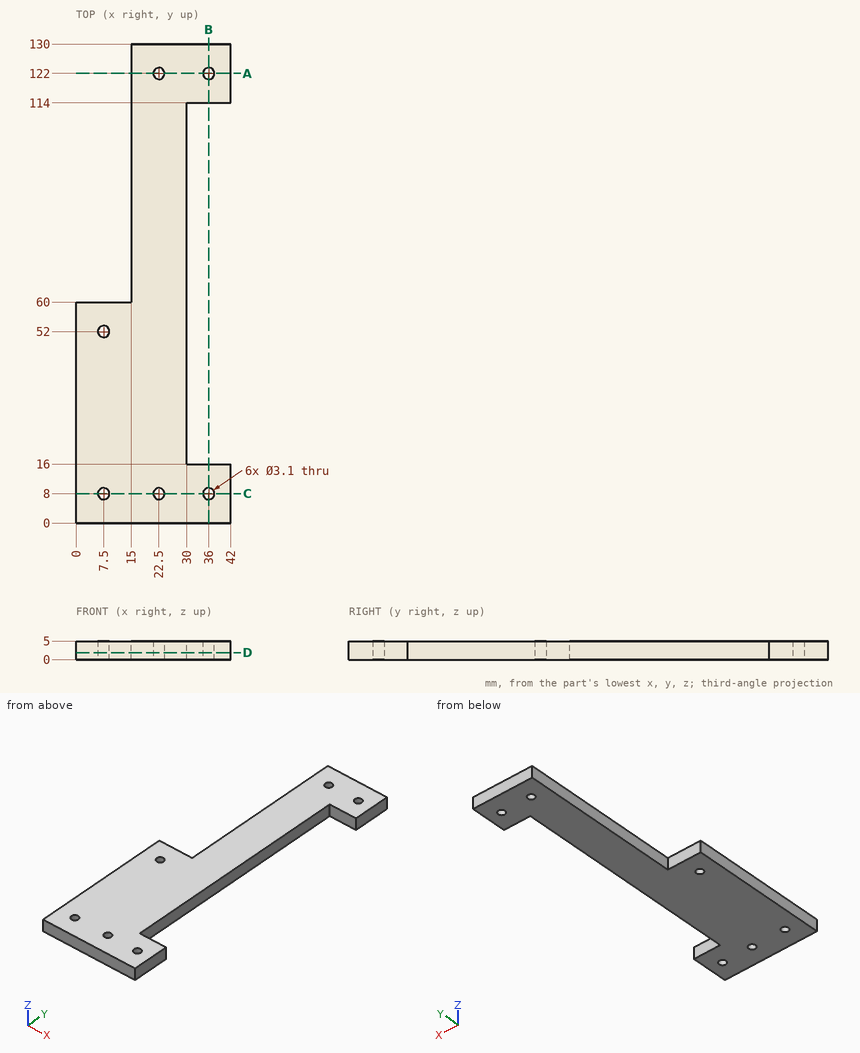
Design review of the part shown in the three views and the two pictorial views. Dimensions are in mm from the part's minimum x, y and z. Coordinates: 2 decimals unless noted, no trailing zeros. Write each loop counter-clockwise with the first axis right and the second up, starting at its lowest first coordinate (ties: lowest second). Pieces come first, ordered by that corner, then holes.
1) We need section B-B on x = 36. State the section outline as (y, z) points, then the cut area to 3 significant figures.
2) We need section C-C on y = 8. State the section outline as (x, z) points, then the cut area to 4 significant figures.
3) To check wall thickness, follow probe 1 along Y at (x, z) = (7.5, 2.15); probe 2 along Y at (x, z) = (22.5, 1.05); probe 3 along Y at (x, z) = (36, 3.8). State the ranges of each line that lie inside material, in increasing order.
4) We need section A-A on y = 122. State the section outline as (x, z) points, then the cut area to 3 significant figures.
5) We need section D-D on z = 1.9. State the section outline as (x, y) points, then the cut area to 3 significant figures.
Answer list:
1. outline: (0, 0) - (6.45, 0) - (6.45, 5) - (0, 5) - close; (9.55, 0) - (16, 0) - (16, 5) - (9.55, 5) - close; (114, 0) - (120.45, 0) - (120.45, 5) - (114, 5) - close; (123.55, 0) - (130, 0) - (130, 5) - (123.55, 5) - close
1. area: 129 mm2
2. outline: (0, 0) - (5.95, 0) - (5.95, 5) - (0, 5) - close; (9.05, 0) - (20.95, 0) - (20.95, 5) - (9.05, 5) - close; (24.05, 0) - (34.45, 0) - (34.45, 5) - (24.05, 5) - close; (37.55, 0) - (42, 0) - (42, 5) - (37.55, 5) - close
2. area: 163.5 mm2
3. probe 1: y = 0 to 6.45, 9.55 to 50.45, 53.55 to 60
3. probe 2: y = 0 to 6.45, 9.55 to 120.45, 123.55 to 130
3. probe 3: y = 0 to 6.45, 9.55 to 16, 114 to 120.45, 123.55 to 130
4. outline: (15, 0) - (20.95, 0) - (20.95, 5) - (15, 5) - close; (24.05, 0) - (34.45, 0) - (34.45, 5) - (24.05, 5) - close; (37.55, 0) - (42, 0) - (42, 5) - (37.55, 5) - close
4. area: 104 mm2
5. outline: (0, 0) - (42, 0) - (42, 16) - (30, 16) - (30, 114) - (42, 114) - (42, 130) - (15, 130) - (15, 60) - (0, 60) - close; hole circle Ø3.1 at (7.5, 8); hole circle Ø3.1 at (7.5, 52); hole circle Ø3.1 at (22.5, 8); hole circle Ø3.1 at (22.5, 122); hole circle Ø3.1 at (36, 8); hole circle Ø3.1 at (36, 122)
5. area: 3,190 mm2
